CAD build for the part. Positions are in the model's coordinates, mm. A direction names the side the tool comes from. Round coordinates to 2 decimals unless told otherwise and drop trailing zeros. Write each loop counter-clockwise with the first axis right and the second up, starting at its lowest first coordinate (ties: lowest second). Pieces come first, ordered by that corner, then holes. Notation, with made-up numbers: (41.25, 8.5) - (48.25, 8.5) arc R22 cw to (48.25, 23.5) - close; hole circle Ø8 at (34, 57.5). An arc over 180 degrees is marked (long way). Use one line per item in the form item = value. Start each with the question number.
Item 1: Band-saw the part on D-D, the plane z = -14.5. List the corners of the cut face in (x, y).
Item 2: Tool access for faces 1 (the cylindrical face through (4.88, -14.79, -1.08)), 2 (the cylindrical face through (21.99, 2.85, -5.28)): list every direction of +Z, -Z, +X, -X, +Y, -Y with a clear straight run to the whole face (end or side of a thin tool).
Item 3: Pin check, flat tips, straight feed: pin 1 (3 mm diameter, centred on x = 0, y = -15, fed in from +Z); pin 2 (8 mm diameter, centred on x = -10.5, z = 9.5, fed in from -Y). Stop position of each tip, or through.
Item 4: Band-saw the part on A-A, the plane z = 0. List the corners of the cut face in (x, y), and give its area (3 significant figures).
Item 5: Band-saw the part on C-C, the plane x = -8. List the corners of the cut face in (y, z).
Item 6: Band-saw the part on B-B, the plane y = 75. List the corners of the cut face in (x, z), and give its area (3 significant figures).
Item 7: Drill centre lines: L1, parallel to Y at x = 15, z = -19; L2, parallel to Y at x = -19, z = -19; L3, parallel to Z at x = 2.5, y = 2.5. Where is each one in solid material? Low to high.
from build123d import *

# Parameters (mm, degrees)
SKETCH1_W           = 50
SKETCH1_H           = 50
BOSS_EXTRUDE1_DEPTH = 100
SKETCH2_R           = 5
BOSS_EXTRUDE2_DEPTH = 30
FILLET1_R           = 10
FILLET2_R           = 10


with BuildPart() as part:
    # Sketch1 → Boss-Extrude1 (new body)
    with BuildSketch(Plane(origin=(0, 0, 0), x_dir=(1, 0, 0), z_dir=(0, 1, 0))):
        Rectangle(SKETCH1_W, SKETCH1_H)
    extrude(amount=BOSS_EXTRUDE1_DEPTH)

    # Sketch2 → Boss-Extrude2 (add)
    with BuildSketch(Plane.XZ):
        with Locations(Location((0, 0, 0), (0, 0, 90))):
            Circle(SKETCH2_R)
    extrude(amount=BOSS_EXTRUDE2_DEPTH)

    # Fillet1
    fillet1_edges = [part.edges().sort_by_distance(p)[0] for p in [
        (0, 100, 25),
        (0, 0, 25),
        (25, 50, 25),
        (-25, 50, 25),
    ]]
    fillet(fillet1_edges, radius=FILLET1_R)

    # Fillet2
    # the kernel refuses this fillet: 10 mm, written as the material it takes off along each edge
    with BuildSketch(Plane(origin=(-15, 90, 15), x_dir=(0, 1, 0), z_dir=(-1, 0, 0))) as fillet2_piece_1_section:
        Polygon((0, 0), (FILLET2_R, 0), (FILLET2_R, -FILLET2_R), (0, -FILLET2_R), align=None)
    fillet2_piece_1 = extrude(amount=FILLET2_R, mode=Mode.PRIVATE)
    fillet2_piece_1 = fillet2_piece_1 - Plane(origin=(-15, 90, 15), x_dir=(0, -0.7071067811865475, -0.7071067811865475), z_dir=(-1, 0, 0)) * Sphere(FILLET2_R, mode=Mode.PRIVATE)
    add(fillet2_piece_1, mode=Mode.SUBTRACT)
    with BuildSketch(Plane(origin=(15, 90, 15), x_dir=(1, 0, 0), z_dir=(0, 1, 0))) as fillet2_piece_2_section:
        Polygon((0, 0), (FILLET2_R, 0), (FILLET2_R, -FILLET2_R), (0, -FILLET2_R), align=None)
    fillet2_piece_2 = extrude(amount=FILLET2_R, mode=Mode.PRIVATE)
    fillet2_piece_2 = fillet2_piece_2 - Plane(origin=(15, 90, 15), x_dir=(-0.7071067811865475, 0, -0.7071067811865475), z_dir=(0, 1, 0)) * Sphere(FILLET2_R, mode=Mode.PRIVATE)
    add(fillet2_piece_2, mode=Mode.SUBTRACT)
    with BuildSketch(Plane(origin=(-15, 10, 15), x_dir=(0, -1, 0), z_dir=(-1, 0, 0))) as fillet2_piece_3_section:
        Polygon((0, 0), (FILLET2_R, 0), (FILLET2_R, FILLET2_R), (0, FILLET2_R), align=None)
    fillet2_piece_3 = extrude(amount=FILLET2_R, mode=Mode.PRIVATE)
    fillet2_piece_3 = fillet2_piece_3 - Plane(origin=(-15, 10, 15), x_dir=(0, 0.7071067811865475, -0.7071067811865475), z_dir=(-1, 0, 0)) * Sphere(FILLET2_R, mode=Mode.PRIVATE)
    add(fillet2_piece_3, mode=Mode.SUBTRACT)
    with BuildSketch(Plane(origin=(15, 10, 15), x_dir=(1, 0, 0), z_dir=(0, -1, 0))) as fillet2_piece_4_section:
        Polygon((0, 0), (FILLET2_R, 0), (FILLET2_R, FILLET2_R), (0, FILLET2_R), align=None)
    fillet2_piece_4 = extrude(amount=FILLET2_R, mode=Mode.PRIVATE)
    fillet2_piece_4 = fillet2_piece_4 - Plane(origin=(15, 10, 15), x_dir=(-0.7071067811865475, 0, -0.7071067811865475), z_dir=(0, -1, 0)) * Sphere(FILLET2_R, mode=Mode.PRIVATE)
    add(fillet2_piece_4, mode=Mode.SUBTRACT)
    with BuildSketch(Plane(origin=(-25, 100, 15), x_dir=(0, -1, 0), z_dir=(0, 0, -1)), Plane(origin=(25, 0, -50), x_dir=(-1, 0, 0), z_dir=(0, 0, 1))) as fillet2_piece_5:
        with BuildLine():
            CenterArc((FILLET2_R, -FILLET2_R), FILLET2_R, 90, 90)
            Line((0, -FILLET2_R), (0, 0))
            Line((0, 0), (FILLET2_R, 0))
        make_face()
    extrude(amount=65, mode=Mode.SUBTRACT)
    with BuildSketch(Plane(origin=(25, 100, -50), x_dir=(-1, 0, 0), z_dir=(0, 0, 1)), Plane(origin=(-25, 0, 15), x_dir=(0, 1, 0), z_dir=(0, 0, -1))) as fillet2_piece_6:
        with BuildLine():
            CenterArc((FILLET2_R, FILLET2_R), FILLET2_R, 180, 90)
            Line((0, FILLET2_R), (0, 0))
            Line((0, 0), (FILLET2_R, 0))
        make_face()
    extrude(amount=65, mode=Mode.SUBTRACT)


solid = part.part
Determined:
q1.outline = (-25, 10) arc R10 ccw to (-15, 0) - (15, 0) arc R10 ccw to (25, 10) - (25, 90) arc R10 ccw to (15, 100) - (-15, 100) arc R10 ccw to (-25, 90) - close
q2.face_1 = -Y
q2.face_2 = +Z, -Z, +X, -Y
q3.pin_1 = 5
q3.pin_2 = 0
q4.outline = (-25, 10) arc R10 ccw to (-15, 0) - (-5, 0) - (-5, -30) - (5, -30) - (5, 0) - (15, 0) arc R10 ccw to (25, 10) - (25, 90) arc R10 ccw to (15, 100) - (-15, 100) arc R10 ccw to (-25, 90) - close
q4.area = 5,210 mm²
q5.outline = (0, -25) - (100, -25) - (100, 15) arc R10 ccw to (90, 25) - (10, 25) arc R10 ccw to (0, 15) - close
q6.outline = (-25, -25) - (25, -25) - (25, 15) arc R10 ccw to (15, 25) - (-15, 25) arc R10 ccw to (-25, 15) - close
q6.area = 2,460 mm²
q7.L1 = 0 to 100
q7.L2 = 0.83 to 99.17
q7.L3 = -25 to 21.61
